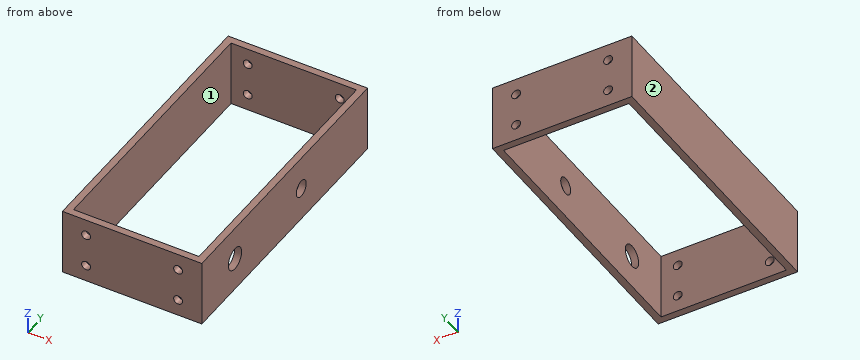
from build123d import *

# Parameters (mm, degrees)
SKETCH_1_W                      = 50
SKETCH_1_H                      = 100
SKETCH_1_W_2                    = 45
SKETCH_1_H_2                    = 95
EXTRUDE_1_DEPTH                 = 24
CUT_EXTRUDE_2_DEPTH             = 106.834776893
CUT_EXTRUDE_2_DEPTH_BACK        = 106.834776893
SKETCH_3_R                      = 1.6
CUT_EXTRUDE_3_REACH             = 76.673
SKETCH_4_R                      = 3
SKETCH_4_R_2                    = 4
CUT_EXTRUDE_3_DIRECTION_2_DEPTH = 75.67261881


with BuildPart() as part:
    # ｽｹｯﾁ1 → ﾎﾞｽ - 押し出し1 (new body)
    with BuildSketch(Plane.XY):
        Rectangle(SKETCH_1_W, SKETCH_1_H)
        Rectangle(SKETCH_1_W_2, SKETCH_1_H_2, mode=Mode.SUBTRACT)
    extrude(amount=EXTRUDE_1_DEPTH)

    # ｽｹｯﾁ3 → ｶｯﾄ - 押し出し2 (cut, two sides: drawn at the far end of the back side and taken through both)
    with BuildSketch(Plane(origin=(0, 50, 0), x_dir=(1, 0, 0), z_dir=(0, 1, 0)).offset(-CUT_EXTRUDE_2_DEPTH_BACK)):
        with Locations(Location((-16.5, -6, 0), (0, 0, 90))):
            Circle(SKETCH_3_R)
        with Locations(Location((16.5, -6, 0), (0, 0, 90))):
            Circle(SKETCH_3_R)
        with Locations(Location((16.5, -18, 0), (0, 0, 90))):
            Circle(SKETCH_3_R)
        with Locations(Location((-16.5, -18, 0), (0, 0, 90))):
            Circle(SKETCH_3_R)
    extrude(amount=CUT_EXTRUDE_2_DEPTH + CUT_EXTRUDE_2_DEPTH_BACK, mode=Mode.SUBTRACT)

    # ｽｹｯﾁ4 → ｶｯﾄ - 押し出し3 (cut, up to next)
    with BuildSketch(Plane(origin=(25, 0, 0), x_dir=(0, 0, -1), z_dir=(1, 0, 0)), mode=Mode.PRIVATE) as cut_extrude_3_sk1:
        with Locations(Location((-12, 10, 0), (0, 0, 270))):
            Circle(SKETCH_4_R)
    cut_extrude_3_tool1 = extrude(cut_extrude_3_sk1.sketch, amount=-CUT_EXTRUDE_3_REACH, mode=Mode.PRIVATE) & part.part
    # ｽｹｯﾁ4 → ｶｯﾄ - 押し出し3 (cut, up to next)
    with BuildSketch(Plane(origin=(25, 0, 0), x_dir=(0, 0, -1), z_dir=(1, 0, 0)), mode=Mode.PRIVATE) as cut_extrude_3_sk2:
        with Locations(Location((-12, -30, 0), (0, 0, 270))):
            Circle(SKETCH_4_R_2)
    cut_extrude_3_tool2 = extrude(cut_extrude_3_sk2.sketch, amount=-CUT_EXTRUDE_3_REACH, mode=Mode.PRIVATE) & part.part
    add(cut_extrude_3_tool1.solids().sort_by_distance((25, 10, 12))[0], mode=Mode.SUBTRACT)
    add(cut_extrude_3_tool2.solids().sort_by_distance((25, -30, 12))[0], mode=Mode.SUBTRACT)

    # ｽｹｯﾁ4 → ｶｯﾄ - 押し出し3 direction 2 (cut)
    with BuildSketch(Plane(origin=(25, 0, 0), x_dir=(0, 0, -1), z_dir=(1, 0, 0))):
        with Locations(Location((-12, 10, 0), (0, 0, 270))):
            Circle(SKETCH_4_R)
        with Locations(Location((-12, -30, 0), (0, 0, 270))):
            Circle(SKETCH_4_R_2)
    extrude(amount=CUT_EXTRUDE_3_DIRECTION_2_DEPTH, mode=Mode.SUBTRACT)


solid = part.part
CAD build for the part. Positions are in the model's coordinates, mm. Face numbers are marked on the shaded views. A direction names the side the tool comes from. Coordinates: 2 decimals unless noted, no trailing zeros. Write each loop counter-clockwise with the first axis right and the second up, starting at its lowest first coordinate (ties: lowest second). Pieces come first, ordered by that corner, then holes. Notation, with made-up numbers: M 65,-26.5 L 101,-26.5 A9 ccw 101,-12.5 Z; hole C 22.25,-14 d11. An arc over 180 degrees is marked long. Answer as a JSON object with one key per item and string values. Group by question number.
1) Tool access for the marked faces 1 and 2: list every direction of +Z, -Z, +X, -X, +Y, -Y with a clear straight run to the whole face (end or side of a thin tool).
2) Saw through at D-D (z = 6). Write the cut outline in (x, y).
3) Saw through at B-B (x = -3). Write the cut outline in (y, z), plus the area to 3 significant figures.
4) Saw through at A-A (y = 33). Write the cut outline in (x, z).
5) Wall check: line 1 (Y direction, x = 23.65, z = 12); line 2 (X direction, y = 48.25, z = 6); line 3 (Y direction, x = 17, z = 20). Give the ranges that are in metal, low to high. Write a range as from..to.
6) Saw through at C-C (z = 12). Write the cut outline in (x, y).
Values follow:
{
 "1": {"face 1": "+Z, -Z", "face 2": "+Z, -Z, -X, +Y, -Y"},
 "2": {"outline": "M -25,-50 L -18.1,-50 L -18.1,-47.5 L -22.5,-47.5 L -22.5,47.5 L -18.1,47.5 L -18.1,50 L -25,50 Z; M -14.9,-50 L 14.9,-50 L 14.9,-47.5 L -14.9,-47.5 Z; M -14.9,47.5 L 14.9,47.5 L 14.9,50 L -14.9,50 Z; M 18.1,-50 L 25,-50 L 25,50 L 18.1,50 L 18.1,47.5 L 22.5,47.5 L 22.5,-47.5 L 18.1,-47.5 Z"},
 "3": {"outline": "M -50,0 L -47.5,0 L -47.5,24 L -50,24 Z; M 47.5,0 L 50,0 L 50,24 L 47.5,24 Z", "area": "120 mm2"},
 "4": {"outline": "M -25,0 L -22.5,0 L -22.5,24 L -25,24 Z; M 22.5,0 L 25,0 L 25,24 L 22.5,24 Z"},
 "5": {"line 1": "y = -50..-34, -26..7, 13..50", "line 2": "x = -25..-18.1, -14.9..14.9, 18.1..25", "line 3": "y = -50..-47.5, 47.5..50"},
 "6": {"outline": "M -25,-50 L 25,-50 L 25,-34 L 22.5,-34 L 22.5,-47.5 L -22.5,-47.5 L -22.5,47.5 L 22.5,47.5 L 22.5,13 L 25,13 L 25,50 L -25,50 Z; M 22.5,-26 L 25,-26 L 25,7 L 22.5,7 Z"}
}
